from build123d import *

# Parameters (mm, degrees)
BOSS_EXTRUDE1_DEPTH = 11
CUT_EXTRUDE1_DEPTH  = 44.327243162
CUT_EXTRUDE2_DEPTH  = 44.327243162
CUT_EXTRUDE3_DEPTH  = 43.793106922


with BuildPart() as part:
    # Sketch1 → Boss-Extrude1 (new body)
    with BuildSketch(Plane(origin=(0, 11, 0), x_dir=(-1, 0, 0), z_dir=(0, 1, 0))):
        with BuildLine():
            Line((-10, 0), (-40, 0))
            Line((-40, 0), (-40, -10.5))
            Line((-40, -10.5), (-32.477225575, -10.5))
            ThreePointArc((-32.477225575, -10.5), (-27, -12.5), (-21.522774425, -10.5))
            Line((-21.522774425, -10.5), (-10, -10.5))
            Line((-10, -10.5), (-10, 0))
        make_face()
    extrude(amount=-BOSS_EXTRUDE1_DEPTH)

    # Sketch2 → Cut-Extrude1 (cut, through all)
    with BuildSketch(Plane.XZ):
        with BuildLine():
            Line((31, 0), (23, 0))
            Line((23, 0), (23, -4))
            ThreePointArc((23, -4), (27, -8), (31, -4))
            Line((31, -4), (31, 0))
        make_face()
    extrude(amount=-CUT_EXTRUDE1_DEPTH, mode=Mode.SUBTRACT)

    # Sketch3 → Cut-Extrude2 (cut, through all)
    with BuildSketch(Plane.XY):
        with BuildLine():
            Line((34.920990299, 4.458012444), (36, 3.340665191))
            Line((36, 3.340665191), (37.079009701, 4.458012444))
            ThreePointArc((37.079009701, 4.458012444), (36, 7), (34.920990299, 4.458012444))
        make_face()
    extrude(amount=-CUT_EXTRUDE2_DEPTH, mode=Mode.SUBTRACT)

    # Sketch4 → Cut-Extrude3 (cut, through all)
    with BuildSketch(Plane(origin=(0, 0, -10.5), x_dir=(-1, 0, 0), z_dir=(0, 0, -1))):
        with BuildLine():
            Line((-16.244261233, 1.75834099), (-13.771383572, 4.31908077))
            ThreePointArc((-13.771383572, 4.31908077), (-13.429402982, 6.164242918), (-14.994261233, 7.2))
            Line((-14.994261233, 7.2), (-17.494261233, 7.2))
            ThreePointArc((-17.494261233, 7.2), (-19.059119484, 6.164242918), (-18.717138893, 4.31908077))
            Line((-18.717138893, 4.31908077), (-16.244261233, 1.75834099))
        make_face()
    extrude(amount=-CUT_EXTRUDE3_DEPTH, mode=Mode.SUBTRACT)


solid = part.part
Verification items for the finished model (mm, model axes). A direction names the side the tool comes from. Coordinates: 2 decimals unless noted, no trailing zeros. Write each loop counter-clockwise with the first axis right and the second up, starting at its lowest first coordinate (ties: lowest second). Pieces come first, ordered by that corner, then holes. Notation, with made-up numbers: M 56.25,-34.75 L 105.25,-34.75 A19 cw 105.25,-9.75 Z; hole C 86,30 d3. An arc over 180 degrees is marked long. Use a Markdown table: item, result.
Q1. Thickness scan on line 1 (X direction, y = 5.5, z = -2.5); line 2 (X direction, y = 0.75, z = -2.25); line 3 (Z direction, x = 36.25, y = 8). Record the ranges inside material, lowest first.
Reply:
| item | result |
|---|---|
| line 1 | x = 10 to 13.29, 19.19 to 23, 31 to 34.5, 37.5 to 40 |
| line 2 | x = 10 to 23, 31 to 40 |
| line 3 | z = -10.5 to 0 |
Q2. Go/stop test with a flat-tipped pin: P1, Ø2.5, axis at x = 35.5, y = 8, coming from the -Z side. Record where the tip stops, or that it passes through.
Reply:
| item | result |
|---|---|
| P1 | stops at z = -10.5 |
Q3. Set-up check for faces 1 (the face through (31, 5, -2)), 2 (the face through (37, 4, -10.5)), 3 (the face through (17.5, 3.06, -5.32)), 4 (the face through (16, 8, -10.5)): record each of +Z, -Z, +X, -X, +Y, -Y from which the full face is reachable in a straight line by a thin tool's end or side.
Reply:
| item | result |
|---|---|
| face 1 | +Z, +Y, -Y |
| face 2 | -Z, +X, +Y, -Y |
| face 3 | +Z, -Z |
| face 4 | -Z, -X, +Y, -Y |
Q4. Draft check along X on faces 5 (the face through (15.025, 3.021, -5.324)), 6 (the face through (40, 6, -5)), 7 (the face through (27.1, 5.6, -12.5)). Enter one of: +X half, -X half, draft (parallel to the pull), parting line (faces both ways), or undercut.
Reply:
| item | result |
|---|---|
| face 5 | undercut |
| face 6 | +X half |
| face 7 | parting line |
Q5. Sectioned sample at B-B, the plane z = -9.25. Record the boundary of the cut face in (x, y), plus the area to 3 significant figures.
Reply:
| item | result |
|---|---|
| outline | M 10,0 L 40,0 L 40,11 L 10,11 Z; hole M 13.77,4.32 L 16.24,1.76 L 18.72,4.32 A1.7 ccw 17.49,7.2 L 14.99,7.2 A1.7 ccw Z; hole M 34.92,4.46 L 36,3.34 L 37.08,4.46 A1.5 ccw long Z |
| area | 301 mm² |
Q6. Sectioned sample at A-A, the plane z = -2.75. Record the boundary of the cut face in (x, y).
Reply:
| item | result |
|---|---|
| outline | M 10,0 L 23,0 L 23,11 L 10,11 Z; M 31,0 L 40,0 L 40,11 L 31,11 Z; hole M 13.77,4.32 L 16.24,1.76 L 18.72,4.32 A1.7 ccw 17.49,7.2 L 14.99,7.2 A1.7 ccw Z; hole M 34.92,4.46 L 36,3.34 L 37.08,4.46 A1.5 ccw long Z |
Q7. Sectioned sample at D-D, the plane y = 8.5. Record the boundary of the cut face in (x, z), plus the area to 3 significant figures.
Reply:
| item | result |
|---|---|
| outline | M 10,-10.5 L 21.52,-10.5 A8.5 ccw 32.48,-10.5 L 40,-10.5 L 40,0 L 31,0 L 31,-4 A4 cw 23,-4 L 23,0 L 10,0 Z |
| area | 273 mm² |
Q8. Sectioned sample at C-C, the plane y = 5.5. Record the boundary of the cut face in (x, z), plus the area to 3 significant figures.
Reply:
| item | result |
|---|---|
| outline | M 10,-10.5 L 13.29,-10.5 L 13.29,0 L 10,0 Z; M 19.19,-10.5 L 21.52,-10.5 A8.5 ccw 32.48,-10.5 L 34.5,-10.5 L 34.5,0 L 31,0 L 31,-4 A4 cw 23,-4 L 23,0 L 19.19,0 Z; M 37.5,-10.5 L 40,-10.5 L 40,0 L 37.5,0 Z |
| area | 179 mm² |
